Geometry: final body of the model. Coordinates: model frame, mm. A direction names the side the tool comes from. Coordinates: 2 decimals unless noted, no trailing zeros. Write each loop counter-clockwise with the first axis right and the second up, starting at its lowest first coordinate (ties: lowest second). Pieces come first, ordered by that corner, then holes.
from build123d import *

# Parameters (mm, degrees)
BOSS_EXTRUDE1_DEPTH = 3.175


with BuildPart() as part:
    # Sketch1 → Boss-Extrude1 (new body)
    with BuildSketch(Plane(origin=(0, 0, 0), x_dir=(1, 0, 0), z_dir=(0, 1, 0))):
        with BuildLine():
            Line((0, 0), (0, 12.7))
            Line((0, 12.7), (-3.175, 12.7))
            Line((-3.175, 12.7), (-3.175, 16.66875))
            ThreePointArc((-3.175, 16.66875), (-0.79375, 19.05), (-3.175, 21.43125))
            Line((-3.175, 21.43125), (-3.175, 25.4))
            Line((-3.175, 25.4), (0, 25.4))
            Line((0, 25.4), (0, 38.1))
            Line((0, 38.1), (38.1, 38.1))
            Line((38.1, 38.1), (38.1, 25.4))
            Line((38.1, 25.4), (41.275, 25.4))
            Line((41.275, 25.4), (41.275, 21.43125))
            ThreePointArc((41.275, 21.43125), (38.89375, 19.05), (41.275, 16.66875))
            Line((41.275, 16.66875), (41.275, 12.7))
            Line((41.275, 12.7), (38.1, 12.7))
            Line((38.1, 12.7), (38.1, 0))
            Line((38.1, 0), (0, 0))
        make_face()
    extrude(amount=BOSS_EXTRUDE1_DEPTH)


solid = part.part
Item 1: Set-up query: faces 5 (the flat face through (0, 2, -32)), 6 (the flat face through (0, 2, -6)), 7 (the flat face through (38.1, 2, -32)). Return all of +Z, -Z, +X, -X, +Y, -Y with unobstructed straight access to the full face (end or side cutting, diameter ignored); none if empty.
Derived:
face 5: -Z, -X, +Y, -Y
face 6: +Z, -X, +Y, -Y
face 7: -Z, +X, +Y, -Y
Item 2: Material intervals for probe 1 along X at (y, z) = (1.5, -30.5); probe 2 along X at (y, z) = (2.1, -20), sorted ascending.
Derived:
probe 1: x = 0 to 38.1
probe 2: x = -0.99 to 39.09
Item 3: Section B-B, the plane z = -19.05. Output: boundary loops of the cut face in (x, y) (3 decimals), plus the area to 3 significant figures.
Derived:
outline: (-0.794, 0) - (38.894, 0) - (38.894, 3.175) - (-0.794, 3.175) - close
area: 126 mm2
Item 4: Pull-direction query (Z, two-part tool) for faces 1 (the cylindrical face through (-0.794, 1.565, -18.998)), 2 (the flat face through (19, 2, 0)), 3 (the flat face through (-3.175, 2, -23)), 4 (the flat face through (19, 2, -38.1)); classes: released by +Z, released by -Z, zero draft, split by the parting line, or undercut.
Derived:
face 1: undercut
face 2: released by +Z
face 3: zero draft
face 4: released by -Z
Item 5: Pin query (flat end, axial travel): pin 1 (1.6 mm diameter, centred on x = 39.5, y = 2, fed in from +Z); pin 2 (1.6 mm diameter, centred on x = 39.5, y = 1, fed in from -Z). Return the tip coordinate at first contact, or that it passes through.
Derived:
pin 1: stops at z = -12.7
pin 2: stops at z = -25.4
Item 6: Section C-C, the plane z = -26.5. Output: boundary loops of the cut face in (x, y) (3 decimals).
Derived:
outline: (0, 0) - (38.1, 0) - (38.1, 3.175) - (0, 3.175) - close
